Geometry: final body of the model. Coordinates: model frame, mm. A direction names the side the tool comes from. Round coordinates to 2 decimals unless told otherwise and drop trailing zeros. Loops run counter-clockwise (first coordinate to the right, second up) from the corner with the lowest first, then second, coordinate; pieces in that order, holes last. Notation, with made-up numbers: (42, 19) -> (93, 19) arc R21 cw to (93, 42) -> close; hole circle Ø11 at (-10, -12). An arc over 180 degrees is marked (long way). Answer in a Markdown table with one row per item.
```python
from build123d import *

# Parameters (mm, degrees)
F0_R      = 8
F1_DEPTH  = 330
F3_DEPTH  = 30
F5_DEPTH  = 20
F6_R      = 12.5
F7_DEPTH  = 57
F8_R      = 3.3
F9_DEPTH  = 43.001
F10_W     = 60
F10_H     = 60
F11_DEPTH = 101
F13_DEPTH = 32.5
F14_W     = 65.58
F14_H     = 3
F15_DEPTH = 65


# Not quite as in the source:
# - a feature names something its author has since deleted; it is built from what else it names


with BuildPart() as f1:
    # F0 (on Right) → F1 (new body)
    with BuildSketch(Plane.YZ):
        Circle(F0_R)
    extrude(amount=F1_DEPTH)

    # F2 (on face) → F3 (join)
    with BuildSketch(Plane.YZ.offset(330)):
        Polygon((30, 7.5), (17, 7.5), (17, 18), (-17, 18), (-17, 7.5), (-30, 7.5), (-30, -25), (30, -25), align=None)
    extrude(amount=-F3_DEPTH)

    # F4 (on face) → F5 (join)
    with BuildSketch(Plane(origin=(0, 0, 0), x_dir=(0, -1, 0), z_dir=(-1, 0, 0))):
        Polygon((17, 7.5), (17, 18), (-17, 18), (-17, 7.5), (-30, 7.5), (-30, -25), (30, -25), (30, 7.5), align=None)
    extrude(amount=-F5_DEPTH)

    # F6 (on face) → F7 (join)
    with BuildSketch(Plane.YZ.offset(330)):
        Circle(F6_R)
    extrude(amount=F7_DEPTH)

    # F8 (on face) → F9 (cut, through all)
    with BuildSketch(Plane.XY.offset(18)):
        with Locations((306, 23)):
            Circle(F8_R)
        with Locations((319, 23)):
            Circle(F8_R)
        with Locations((306, -23)):
            Circle(F8_R)
        with Locations((319, -23)):
            Circle(F8_R)
        with Locations((10, 23)):
            Circle(F8_R)
        with Locations((10, -23)):
            Circle(F8_R)
    extrude(amount=-F9_DEPTH, mode=Mode.SUBTRACT)

    # F10 (on face) → F11 (join)
    with BuildSketch(Plane.YZ.offset(387)):
        Rectangle(F10_W, F10_H)
    extrude(amount=F11_DEPTH)

    # F12 (on Front) → F13 (join, symmetric)
    with BuildSketch(Plane.XZ):
        Polygon((387, 30), (384, 30), (384, -38.58), (452.58, -38.58), (452.58, -35.58), (387, -35.58), align=None)
    extrude(amount=F13_DEPTH, both=True)

    # F14 (on face) → F15 (join, through all)
    with BuildSketch(Plane.XZ.offset(32.5)):
        with Locations((351.21, -37.08)):
            Rectangle(F14_W, F14_H)
    extrude(amount=-F15_DEPTH)


solid = f1.part
```
Item 1: Mould query, pull axis X, two halves, no side actions, for faces 1 (the flat face through (0, 0, -3)), 2 (the flat face through (20, 7, -8)), 3 (the flat face through (385, -32.5, -19)). Classes: released by +X, released by -X, zero draft, split by the parting line, or undercut.
Ans:
| item | result |
|---|---|
| face 1 | released by -X |
| face 2 | undercut |
| face 3 | zero draft |
Item 2: Section query D-D, the plane x = 184. Output: boundary loops of the cut face in (y, z), and give its area (3 significant figures).
Ans:
| item | result |
|---|---|
| outline | circle Ø16 at (0, 0) |
| area | 201 mm2 |
Item 3: First-contact query: P1, Ø11.5, axis at x = 7, z = 14, coming from the -Y side; P2, Ø22, axis at x = 9.5, y = 4, coming from the +Z side; P3, Ø16, axis at x = 13.5, y = 4, coming from the -Z side. Flat tips, straight axial feed; report the tip coordinate or a pass-through.
Ans:
| item | result |
|---|---|
| P1 | y = -17 |
| P2 | z = 18 |
| P3 | z = -25 |
Item 4: Ray query, L1, parallel to X at y = 1, z = -22.5; L2, parallel to Y at x = 10, z = -7; L3, parallel to Z at x = 452.5, y = 14.5. Return the intervals inside material, ascending.
Ans:
| item | result |
|---|---|
| L1 | 0 to 20, 300 to 330, 384 to 488 |
| L2 | -30 to -26.3, -19.7 to 19.7, 26.3 to 30 |
| L3 | -38.58 to -35.58, -30 to 30 |
Item 5: Section query A-A, the plane x = 348. Output: boundary loops of the cut face in (y, z).
Ans:
| item | result |
|---|---|
| outline | (-32.5, -38.58) -> (32.5, -38.58) -> (32.5, -35.58) -> (-32.5, -35.58) -> close; circle Ø25 at (0, 0) |
Item 6: Section query B-B, the plane y = 0. Output: boundary loops of the cut face in (x, z), and give its area (3 significant figures).
Ans:
| item | result |
|---|---|
| outline | (0, -25) -> (20, -25) -> (20, -8) -> (300, -8) -> (300, -25) -> (330, -25) -> (330, -12.5) -> (384, -12.5) -> (384, -35.58) -> (318.42, -35.58) -> (318.42, -38.58) -> (452.58, -38.58) -> (452.58, -35.58) -> (387, -35.58) -> (387, -30) -> (488, -30) -> (488, 30) -> (384, 30) -> (384, 12.5) -> (330, 12.5) -> (330, 18) -> (300, 18) -> (300, 8) -> (20, 8) -> (20, 18) -> (0, 18) -> close |
| area | 14,600 mm2 |
Item 7: Section query C-C, the plane x = 442. Output: boundary loops of the cut face in (y, z).
Ans:
| item | result |
|---|---|
| outline | (-32.5, -38.58) -> (32.5, -38.58) -> (32.5, -35.58) -> (-32.5, -35.58) -> close; (-30, -30) -> (30, -30) -> (30, 30) -> (-30, 30) -> close |
Item 8: Set-up query: faces 4 (the flat face through (9.9, -26.5, 7.5)), 5 (the flat face through (8, 26, 7.5)), 6 (the flat face through (315, 0, -25)), 7 (the flat face through (315, 0, 18)). Return all of +Z, -Z, +X, -X, +Y, -Y with unobstructed straight access to the full face (end or side cutting, diameter ignored); none if empty.
Ans:
| item | result |
|---|---|
| face 4 | +Z, -X, -Y |
| face 5 | +Z, -X, +Y |
| face 6 | -X, +Y, -Y |
| face 7 | +Z, -X, +Y, -Y |
